Autodesk Inventor part; units mm, degrees
ref_plane "YZ Plane" through (0, 0, 0) normal (1, 0, 0) x (0, 1, 0)
ref_plane "XZ Plane" through (0, 0, 0) normal (0, 1, 0) x (-1, 0, 0)
ref_plane "XY Plane" through (0, 0, 0) normal (0, 0, 1) x (1, 0, 0)
sketch "Sketch1" plane through (0, 0, 0) normal (0, 1, 0) x (-1, 0, 0)
  line L0 (-40, -47.5) -> (40, -47.5)
  line L1 (40, -47.5) -> (40, 47.5)
  line L2 (40, 47.5) -> (-40, 47.5)
  line L3 (-40, 47.5) -> (-40, -47.5)
  line L4 (-40, -47.5) -> (40, 47.5) construction
  line L5 (40, -47.5) -> (-40, 47.5) construction
  point P0 (0, 0)
  dimension "d0" = 80
  dimension "d1" = 95
extrude "Extrusion1" add sketch "Sketch1" along normal blind 8
sketch "Sketch2" plane through (40, 0, 47.5) normal (1, 0, 0) x (0, 0, -1)
  line L0 (0, 0) -> (95, 0)
  line L1 (95, 0) -> (95, 8)
  line L2 (0, 8) -> (95, 8)
  line L3 (0, 0) -> (0, 8)
  line L4 (95, 0) -> (0, 0)
  line L5 (0, 0) -> (0, -16)
  line L6 (2, -18) -> (19.1716, -18)
  line L7 (2, -2) -> (2, -14)
  line L8 (4, -16) -> (17.1716, -16)
  line L9 (20.5858, -17.4142) -> (37.4142, -0.5858)
  line L10 (18.5858, -15.4142) -> (30.5858, -3.4142)
  arc A0 (2, -14) -> (4, -16) centre (4, -14) ccw
  arc A1 (0, -16) -> (2, -18) centre (2, -16) ccw
  arc A2 (19.1716, -18) -> (20.5858, -17.4142) centre (19.1716, -16) ccw
  arc A3 (17.1716, -16) -> (18.5858, -15.4142) centre (17.1716, -14) ccw
  line L11 (4, 0) -> (29.1716, 0)
  arc A4 (30.5858, -3.4142) -> (29.1716, 0) centre (29.1716, -2) ccw
  line L12 (38.8284, 0) -> (47.5, 0)
  arc A5 (38.8284, 0) -> (37.4142, -0.5858) centre (38.8284, -2) ccw
  arc A6 (4, 0) -> (2, -2) centre (4, -2) ccw
  point P0 (0, -18)
  point P1 (20, -18)
  point P2 (22, -16)
  point P3 (38, 0)
  point P4 (34, 0)
  point P5 (34, 0)
  dimension "d4" = 18
  dimension "d5" = 20
  dimension "d6" = 2
  dimension "d7" = 45
  dimension "d8" = 2
  dimension "d9" = 2
  dimension "d10" = 2
extrude "Extrusion2" add sketch "Sketch2" against normal up to surface (80 mm away) contours L0 A6 L7 A0 L8 A3 L10 A4 A5 L9 A2 L6 A1 L5
sketch "Sketch3" plane through (-40, 8, 47.5) normal (0, 0, 1) x (1, 0, 0)
  line L0 (80, 0) -> (0, 0)
  line L1 (0, 0) -> (15, 0)
  line L2 (80, 0) -> (65, 0)
  line L3 (80, -26) -> (0, -26)
  line L4 (15, 0) -> (65, 0)
  line L5 (65, 0) -> (65, -26)
  line L6 (65, -26) -> (15, -26)
  line L7 (15, -26) -> (15, 0)
  line L8 (15, 0) -> (65, 0)
  line L9 (65, 0) -> (65, -8)
  line L10 (65, -8) -> (15, -8)
  line L11 (15, -8) -> (15, 0)
  line L12 (80, -24) -> (80, 0)
  point P0 (40, -8)
  dimension "d13" = 15
  dimension "d15" = 50
  dimension "d16" = 8
  dimension "d41" = 15
extrude "Extrusion3" cut sketch "Sketch3" against normal blind 39 contours L5 L3 L7 L10
sketch "Sketch4" plane through (0, 8, 0) normal (0, 1, 0) x (1, 0, 0)
  line L0 (40, 47.5) -> (-40, 47.5)
  line L1 (-40, 47.5) -> (-40, -47.5)
  line L2 (-40, -47.5) -> (40, -47.5)
  line L3 (40, -47.5) -> (40, 47.5)
  line L4 (40, 47.5) -> (-40, 47.5)
  line L5 (-40, -47.5) -> (-35, -47.5)
  line L6 (-35, -47.5) -> (-35, 47.5)
  line L7 (-35, 47.5) -> (-40, 47.5)
  line L8 (-40, 47.5) -> (-40, -47.5)
  line L9 (40, -47.5) -> (35, -47.5)
  line L10 (35, -47.5) -> (35, 47.5)
  line L11 (35, 47.5) -> (40, 47.5)
  line L12 (40, 47.5) -> (40, -47.5)
  line L13 (40, -47.5) -> (32, -47.5)
  line L14 (32, -47.5) -> (32, -39.5)
  line L15 (32, -39.5) -> (40, -39.5)
  line L16 (40, -39.5) -> (40, -47.5)
  line L17 (-40, -47.5) -> (-32, -47.5)
  line L18 (-32, -47.5) -> (-32, -39.5)
  line L19 (-32, -39.5) -> (-40, -39.5)
  line L20 (-40, -39.5) -> (-40, -47.5)
  line L21 (-40, 47.5) -> (-40, -47.5)
  line L22 (-40, 47.5) -> (-32, 47.5)
  line L23 (-32, 47.5) -> (-32, 39.5)
  line L24 (-32, 39.5) -> (-40, 39.5)
  line L25 (-40, 39.5) -> (-40, 47.5)
  line L26 (40, 47.5) -> (32, 47.5)
  line L27 (32, 47.5) -> (32, 39.5)
  line L28 (32, 39.5) -> (40, 39.5)
  line L29 (40, 39.5) -> (40, 47.5)
  point P0 (0, 0)
  dimension "d19" = 5
  dimension "d20" = 5
  dimension "d21" = 8
  dimension "d22" = 8
  dimension "d23" = 8
  dimension "d24" = 8
  dimension "d25" = 8
  dimension "d26" = 8
  dimension "d27" = 8
  dimension "d28" = 8
extrude "Extrusion4" add sketch "Sketch4" along normal blind 10 contours L3 L28 L10 L0 | L3 L15 L10 L28 | L3 L2 L10 L15 | L6 L24 L1 L0 | L6 L19 L1 L24 | L6 L2 L1 L19
sketch "Sketch6" plane through (0, 8, 0) normal (0, 1, 0) x (1, 0, 0)
  line L0 (40, 47.5) -> (-40, 47.5)
  line L1 (-40, 47.5) -> (-32, 47.5)
  line L2 (-32, 47.5) -> (-32, 39.5)
  line L3 (-32, 39.5) -> (-40, 39.5)
  line L4 (-40, 39.5) -> (-40, 47.5)
  line L5 (40, 47.5) -> (32, 47.5)
  line L6 (32, 47.5) -> (32, 39.5)
  line L7 (32, 39.5) -> (40, 39.5)
  line L8 (40, 39.5) -> (40, 47.5)
  line L9 (-25, -47.5) -> (-40, -47.5)
  line L10 (-40, -47.5) -> (-32, -47.5)
  line L11 (-32, -47.5) -> (-32, -39.5)
  line L12 (-32, -39.5) -> (-40, -39.5)
  line L13 (-40, -39.5) -> (-40, -47.5)
  line L14 (40, -43.5) -> (40, -18.3284)
  line L15 (-35, -47.5) -> (35, -47.5)
  line L16 (40, -40.5) -> (48.82, -40.5) construction
  line L17 (40, -47.5) -> (32, -47.5)
  line L18 (32, -47.5) -> (32, -35.5)
  line L19 (32, -35.5) -> (40, -35.5)
  line L20 (40, -35.5) -> (40, -47.5)
  line L21 (35, -47.5) -> (35, 47.5)
  line L22 (35, -47.5) -> (40, -38.8397)
  line L23 (40, -30.3284) -> (40, -43.5)
  line L24 (35, -47.5) -> (45, -47.5) construction
  point P0 (0, 0)
  dimension "d42" = 8
  dimension "d43" = 8
  dimension "d44" = 8
  dimension "d45" = 8
  dimension "d46" = 8
  dimension "d47" = 8
  dimension "d81" = 8
  dimension "d82" = 12
  dimension "d83" = 60
extrude "Extrusion5" add sketch "Sketch6" along normal blind 100
sketch "Sketch7" plane through (0, 108, 0) normal (0, 1, 0) x (1, 0, 0)
  line L0 (-40, -47.5) -> (-40, -45.5)
  line L1 (-32, 47.5) -> (-40, 47.5)
  line L2 (-40, -47.5) -> (-32, -47.5)
  line L3 (-32, -47.5) -> (-32, 47.5)
  line L4 (-32, 47.5) -> (-40, 47.5)
  line L5 (-40, 47.5) -> (-40, -47.5)
  line L6 (35, -39.5) -> (40, -39.5)
  line L7 (-40, -47.5) -> (40, -47.5)
  line L8 (40, -47.5) -> (40, -39.5)
  line L9 (40, -39.5) -> (-40, -39.5)
  line L10 (-40, -39.5) -> (-40, -47.5)
  line L11 (32, 39.5) -> (32, 47.5)
  line L12 (32, 47.5) -> (40, 47.5)
  line L13 (40, 47.5) -> (40, -47.5)
  line L14 (40, -47.5) -> (32, -47.5)
  line L15 (32, -47.5) -> (32, 47.5)
  point P0 (0, 0)
extrude "Extrusion6" add sketch "Sketch7" along normal blind 8
sketch "Sketch8" plane through (40, 0, -47.5) normal (0, 0, -1) x (-1, 0, 0)
  line L0 (8, 8) -> (72, 8)
  line L1 (8, 8) -> (8, 116)
  line L2 (0, 116) -> (8, 116)
  line L3 (0, 0) -> (0, 116)
  line L4 (0, 0) -> (80, 0)
  line L5 (80, 0) -> (80, 116)
  line L6 (72, 116) -> (80, 116)
  line L7 (72, 8) -> (72, 116)
  line L8 (0, 116) -> (8, 116)
  line L9 (8, 8) -> (8, 108)
  line L10 (0, 116) -> (8, 116)
  line L11 (8, 108) -> (0, 108)
  line L12 (0, 108) -> (0, 116)
  line L13 (0, 108) -> (8, 108)
  line L14 (8, 108) -> (8, 111)
  line L15 (8, 8) -> (8, 116)
  line L16 (8, 111) -> (4, 111)
  line L17 (4, 111) -> (4, 114)
  line L18 (4, 114) -> (8, 114)
  line L19 (80, 116) -> (0, 116)
  line L20 (40, 116) -> (40, 8)
  line L21 (72, 8) -> (8, 8)
  line L22 (80, 116) -> (72, 116)
  line L23 (80, 116) -> (72, 116)
  line L24 (80, 116) -> (72, 116)
  line L25 (72, 108) -> (80, 108)
  line L26 (80, 108) -> (80, 116)
  line L27 (80, 108) -> (72, 108)
  line L28 (72, 108) -> (72, 111)
  line L29 (72, 111) -> (76, 111)
  line L30 (76, 111) -> (76, 114)
  line L31 (76, 114) -> (72, 114)
  line L32 (8, 114) -> (72, 114)
  line L33 (72, 111) -> (8, 111)
  line L34 (72, 114) -> (76, 114)
  line L35 (76, 114) -> (76, 111)
  line L36 (76, 111) -> (72, 111)
  line L37 (72, 116) -> (72, 114)
  line L38 (72, 111) -> (72, 108)
  line L39 (8, 116) -> (8, 114)
  line L40 (8, 111) -> (8, 108)
  line L41 (4, 114) -> (8, 114)
  line L42 (4, 111) -> (8, 111)
  line L43 (4, 114) -> (76, 114)
  line L44 (76, 114) -> (76, 111)
  line L45 (76, 111) -> (4, 111)
  line L46 (4, 111) -> (4, 114)
  point P0 (40, 0)
  dimension "d52" = 3
  dimension "d53" = 4
  dimension "d54" = 3
extrude "Extrusion7" cut sketch "Sketch8" against normal blind 91 contours L33 L1 L32 L20 | L20 L32 L7 L33 | L16 L17 L18 L1 | L7 L31 L30 L29
sketch "Sketch9" plane through (0, 8, 0) normal (0, 1, 0) x (1, 0, 0)
  line L0 (0, -31.5) -> (8.5, -31.5)
  circle A0 centre (8.5, -31.5) radius 2.5
  circle A1 centre (-19.5, -31.5) radius 2.5
  circle A2 centre (-19.5, -31.5) radius 2.5
  line L1 (0, -31.5) -> (-19.5, -31.5)
  line L2 (0, 0) -> (0, -31.5)
  line L3 (0, 0) -> (0, 17.5)
  line L4 (0, 17.5) -> (0, 19)
  line L5 (0, 19) -> (24, 19)
  circle A3 centre (24, 19) radius 2.5
  line L6 (0, 0) -> (2.25, 0)
  line L7 (-27.5, 38.25) -> (28.5, 38.25)
  line L8 (28.5, 38.25) -> (28.5, -36.75)
  line L9 (28.5, -36.75) -> (-27.5, -36.75)
  line L10 (-27.5, -36.75) -> (-27.5, 38.25)
  line L11 (-27.5, 38.25) -> (28.5, -36.75) construction
  line L12 (28.5, 38.25) -> (-27.5, -36.75) construction
  line L13 (-19.5, -31.5) -> (-19.5, -36.75)
  line L14 (25.5, 17) -> (28.5, 17)
  line L15 (28.5, 17) -> (28.5, -36.75)
  point P0 (0.5, 0.75)
  dimension "d63" = 5
  dimension "d61" = 5
  dimension "d62" = 5
  dimension "d64" = 17.5
  dimension "d65" = 8.5
  dimension "d66" = 19.5
  dimension "d67" = 31.5
  dimension "d68" = 24
  dimension "d69" = 43.5
  dimension "d70" = 2.25
  dimension "d71" = 56
  dimension "d72" = 75
  dimension "d73" = 5.25
  dimension "d74" = 3
extrude "Extrusion8" cut sketch "Sketch9" against normal blind 10 contours A0 | L1 L13 A1 | A1 L13 L1 | A3
properties part number "Base"
Work out the finished part from the listing and answer in its coordinate system (mm). A direction names the side the tool comes from. Give positions to 0.01 mm unless a question says otherwise; leave off trailing zeros. Order: outer loops, then holes, each group sorted by start corner. A loop starts at its lowest first (then second) coordinate and runs counter-clockwise, first axis right, second up. Notation, with made-up numbers: (51.25, 86.25) -> (76.25, 86.25) arc R26 cw to (76.25, 108.25) -> close; hole circle Ø11 at (82, 79). An arc over 180 degrees is marked (long way). One line per item, written item: value.
Item 1: Straight lines are drawn through the part: probe 1 along X at (y, z) = (5, 31.5); probe 2 along Z at (x, y) = (24, 4); probe 3 along Y at (x, z) = (33.5, -29.5). For each, find the intervals that lie inside material, in ascending order.
Answer sheet:
probe 1: -40 to -22, -17 to 6, 11 to 40
probe 2: -47.5 to -21.5, -16.5 to 47.5
probe 3: 0 to 8, 108 to 111, 114 to 116
Item 2: A tool of negligible diameter and unlimited length cuts with its end or side. For faces 1 (the flat face through (25, -14, 27)), 2 (the flat face through (-32.2, 111, 7.9)), 3 (the flat face through (-32, -18, 37)), 4 (the flat face through (32.6, -9.5, 23)), from which of +Z, -Z, +X, -X, +Y, -Y can it reach the whole face along a straight path? Write none if from no direction.
Answer sheet:
face 1: +Z, -Z, -Y
face 2: -Z
face 3: +Z, -Z, +X, -X, -Y
face 4: +X, -X
Item 3: Find section D-D, the plane x = 8.5. Give the vertices of the cut face in (y, z), plus the area to 3 significant figures.
Answer sheet:
outline: (0, -47.5) -> (8, -47.5) -> (8, 29) -> (0, 29) -> close; (0, 34) -> (8, 34) -> (8, 47.5) -> (0, 47.5) -> close; (108, 39.5) -> (111, 39.5) -> (111, 43.5) -> (114, 43.5) -> (114, 39.5) -> (116, 39.5) -> (116, 47.5) -> (108, 47.5) -> close
area: 772 mm²
Item 4: Find section A-A, the plane x = 30. Give the vertices of the cut face in (y, z), plus the area to 3 significant figures.
Answer sheet:
outline: (-18, 28.33) arc R2 ccw to (-17.41, 26.91) -> (-0.59, 10.09) arc R2 cw to (0, 8.67) -> (0, -47.5) -> (8, -47.5) -> (8, 47.5) -> (-16, 47.5) arc R2 ccw to (-18, 45.5) -> close; (108, 39.5) -> (111, 39.5) -> (111, 43.5) -> (114, 43.5) -> (114, 39.5) -> (116, 39.5) -> (116, 47.5) -> (108, 47.5) -> close; hole (-16, 30.33) arc R2 ccw to (-15.41, 28.91) -> (-3.41, 16.91) arc R2 ccw to (0, 18.33) -> (0, 43.5) arc R2 ccw to (-2, 45.5) -> (-14, 45.5) arc R2 ccw to (-16, 43.5) -> close
area: 956 mm²
Item 5: Determine the mould class of faces 5 (the flat face through (32.2, 114, 7.9)), 6 (the flat face through (33, -18, 37)), 7 (the flat face through (0, 109, 39.5)) for opening direction Y: released by +Y, released by -Y, zero draft, split by the parting line, or undercut.
Answer sheet:
face 5: undercut
face 6: released by -Y
face 7: zero draft
Item 6: Flat-ended cylindrical pins translate along their axes: P1, Ø4, axis at x = 24, z = -19, coming from the +Y side; P2, Ø5, axis at x = -8.5, z = 2, coming from the -Y side; P3, Ø13, axis at x = 32.5, y = -8, coming from the -Z side; P4, Ø8, axis at x = -14, z = 24, coming from the +Y side. Find the tip coordinate at first contact, or state that the pin passes through.
Answer sheet:
P1: through
P2: y = 0
P3: z = 11
P4: y = 8
Item 7: Find section B-B, the plane z = -19. Give the vertices of the cut face in (x, y).
Answer sheet:
outline: (-40, 0) -> (21.5, 0) -> (21.5, 8) -> (-35, 8) -> (-35, 18) -> (-40, 18) -> close; (-40, 108) -> (-32, 108) -> (-32, 111) -> (-36, 111) -> (-36, 114) -> (-32, 114) -> (-32, 116) -> (-40, 116) -> close; (26.5, 0) -> (40, 0) -> (40, 18) -> (35, 18) -> (35, 8) -> (26.5, 8) -> close; (32, 108) -> (40, 108) -> (40, 116) -> (32, 116) -> (32, 114) -> (36, 114) -> (36, 111) -> (32, 111) -> close
Item 8: Find section C-C, the plane y = 49.5. Give the vertices of the cut face in (x, z), plus the area to 3 significant figures.
Answer sheet:
outline: (-40, -47.5) -> (-32, -47.5) -> (-32, -39.5) -> (-40, -39.5) -> close; (-40, 39.5) -> (-32, 39.5) -> (-32, 47.5) -> (-40, 47.5) -> close; (32, -47.5) -> (40, -47.5) -> (40, -39.5) -> (32, -39.5) -> close; (32, 35.5) -> (40, 35.5) -> (40, 47.5) -> (32, 47.5) -> close
area: 288 mm²
